Design review of the part built by this model. Coordinates are the model's own, in mm. A direction names the side the tool comes from. Round coordinates to 2 decimals unless told otherwise and drop trailing zeros. Loops run counter-clockwise (first coordinate to the right, second up) from the corner with the lowest first, then second, coordinate; pieces in that order, holes last. Notation, with made-up numbers: (-3, -36.75) - (41, -36.75) arc R29 ccw to (41, -13.75) - close; hole circle Ø8 at (22, -37.75). An arc over 180 degrees is marked (long way). Return JSON: item names as keys, results as strings. Group by question number.
from build123d import *

# Parameters (mm, degrees)
F0_W      = 152.4
F0_H      = 101.6
F1_DEPTH  = 12.7
F2_W      = 139.7
F2_H      = 88.9
F3_DEPTH  = 5.08
F4_R      = 5.08
F5_W      = 2.54
F5_H      = 38.1
F6_DEPTH  = 5.08
F7_W      = 2.54
F7_H      = 38.1
F8_DEPTH  = 5.08
F9_W      = 12.7
F9_H      = 12.7
F10_DEPTH = 50.8


with BuildPart() as f1:
    # F0 (on Front) → F1 (new body, symmetric)
    with BuildSketch(Plane.XZ):
        Rectangle(F0_W, F0_H)
    extrude(amount=F1_DEPTH, both=True)

    # F2 (on face) → F3 (cut)
    with BuildSketch(Plane.XZ.offset(12.7)):
        Rectangle(F2_W, F2_H)
    extrude(amount=-F3_DEPTH, mode=Mode.SUBTRACT)

    # F4
    f4_edges = [f1.edges().sort_by_distance(p)[0] for p in [
        (-69.85, -10.16, -44.45),
        (69.85, -10.16, -44.45),
        (69.85, -10.16, 44.45),
        (-69.85, -10.16, 44.45),
        (-76.2, 0, 50.8),
        (-76.2, 0, -50.8),
        (76.2, 0, 50.8),
        (76.2, 0, -50.8),
    ]]
    fillet(f4_edges, radius=F4_R)

    # F5 (on face) → F6 (cut)
    with BuildSketch(Plane.YZ.offset(-69.85)):
        with Locations((-8.89, 0)):
            Rectangle(F5_W, F5_H)
    extrude(amount=-F6_DEPTH, mode=Mode.SUBTRACT)

    # F7 (on face) → F8 (cut)
    with BuildSketch(Plane(origin=(69.85, 0, 0), x_dir=(0, -1, 0), z_dir=(-1, 0, 0))):
        with Locations((8.89, 0)):
            Rectangle(F7_W, F7_H)
    extrude(amount=-F8_DEPTH, mode=Mode.SUBTRACT)

    # F9 (on face) → F10 (join)
    with BuildSketch(Plane(origin=(0, 12.7, 0), x_dir=(-1, 0, 0), z_dir=(0, 1, 0))):
        with Locations((64.77, 39.37)):
            Rectangle(F9_W, F9_H)
        with Locations((64.77, -39.37)):
            Rectangle(F9_W, F9_H)
        with Locations((-64.77, 39.37)):
            Rectangle(F9_W, F9_H)
        with Locations((-64.77, -39.37)):
            Rectangle(F9_W, F9_H)
    extrude(amount=F10_DEPTH)


solid = f1.part
Q1. Add section D-D, the plane z = -12.5. State the section outline as (x, y) points, plus the area to 3 significant figures.
Q2. Draft analysis for pull direction X (two halves, no side actions). For faces 1 (the flat face through (-65, 63.5, -39)), 2 (the flat face through (-58.42, 38, 39)), 3 (the cylindrical face through (75, 0, -49)), state which applies: pulls with the +X half, pulls with the -X half, needs draft (parallel to the pull), parting line crosses it, or undercut.
Q3. Insertion check: pin 1 Ø12 at (y, z) = (24.5, -4.5) entering from +X; pin 2 Ø10 at (x, y) = (-67, 38.5) entering from -Z; pin 3 Ø6.5 at (y, z) = (36.5, 39) entering from -X; pin 4 Ø1.5 at (x, z) = (-5, 9.5) entering from +Y. Each pin has a flat end and moves straight along its axis. Give the tip position at first contact, or say it passes through.
Q4. Add section A-A, the plane y = 52. State the section outline as (x, z) points, plus the area to 3 significant figures.
Q5. For line 1 (Z direction, x = -32, y = -8.5); line 2 (Z direction, x = -60, y = 54.5); line 3 (Y direction, x = -13.5, z = -3.5), list the stretches that pass through material, from the lowest coordinate up.
Q6. Add section B-B, the plane z = -30. State the section outline as (x, y) points, plus the area to 3 significant figures.
Q7. Add section C-C, the plane x = -9. State the section outline as (y, z) points.
Q8. Tool access review of faces 4 (the cylindrical face through (-68.322, -10.124, 43.001)), 5 (the flat face through (58.42, 38, 39)), 6 (the flat face through (-71.12, 38, 39)), 7 (the flat face through (65, 38, -33.02)), 8 (the flat face through (72, -10.16, 0)): name each direction out of +Z, -Z, +X, -X, +Y, -Y from which nothing blocks a thin tool from reaching the whole face with its end or side.
Evaluation:
{
 "1": {"outline": "(-76.2, -12.7) - (-69.85, -12.7) - (-69.85, -10.16) - (-74.93, -10.16) - (-74.93, -7.62) - (74.93, -7.62) - (74.93, -10.16) - (69.85, -10.16) - (69.85, -12.7) - (76.2, -12.7) - (76.2, 12.7) - (-76.2, 12.7) - close", "area": "3,140 mm²"},
 "2": {"face 1": "needs draft", "face 2": "undercut", "face 3": "pulls with the +X half"},
 "3": {"pin 1": "through", "pin 2": "z = -45.72", "pin 3": "x = -71.12", "pin 4": "y = 12.7"},
 "4": {"outline": "(-71.12, -45.72) - (-58.42, -45.72) - (-58.42, -33.02) - (-71.12, -33.02) - close; (-71.12, 33.02) - (-58.42, 33.02) - (-58.42, 45.72) - (-71.12, 45.72) - close; (58.42, -45.72) - (71.12, -45.72) - (71.12, -33.02) - (58.42, -33.02) - close; (58.42, 33.02) - (71.12, 33.02) - (71.12, 45.72) - (58.42, 45.72) - close", "area": "645 mm²"},
 "5": {"line 1": "-50.8 to -44.45, 44.45 to 50.8", "line 2": "-45.72 to -33.02, 33.02 to 45.72", "line 3": "-7.62 to 12.7"},
 "6": {"outline": "(-76.2, -12.7) - (-69.85, -12.7) - (-69.85, -7.62) - (69.85, -7.62) - (69.85, -12.7) - (76.2, -12.7) - (76.2, 12.7) - (-76.2, 12.7) - close", "area": "3,160 mm²"},
 "7": {"outline": "(-12.7, -50.8) - (12.7, -50.8) - (12.7, 50.8) - (-12.7, 50.8) - (-12.7, 44.45) - (-7.62, 44.45) - (-7.62, -44.45) - (-12.7, -44.45) - close"},
 "8": {"face 4": "-Y", "face 5": "+Z, -Z, +Y", "face 6": "+Z, -Z, -X, +Y", "face 7": "+X, -X, +Y", "face 8": "none"}
}
